Autodesk Inventor part; units mm, degrees
ref_plane "YZ Plane" through (0, 0, 0) normal (1, 0, 0) x (0, 1, 0)
ref_plane "XZ Plane" through (0, 0, 0) normal (0, 1, 0) x (-1, 0, 0)
ref_plane "XY Plane" through (0, 0, 0) normal (0, 0, 1) x (1, 0, 0)
sketch "Sketch1" plane through (0, 0, 0) normal (0, 1, 0) x (-1, 0, 0)
  line L0 (0, 0) -> (161, 0)
  line L1 (161, 0) -> (161, -140)
  line L2 (161, -140) -> (0, -140)
  line L3 (0, -140) -> (0, 0)
  line L4 (156, -135) -> (156, -5)
  line L5 (156, -5) -> (5, -5)
  line L6 (5, -5) -> (5, -135)
  line L7 (5, -135) -> (156, -135)
  dimension "d28" = 151
  dimension "d29" = 130
  dimension "d30" = 5
extrude "Extrusion1" add sketch "Sketch1" along normal blind 44.45
sketch "Sketch2" plane through (0, 0, 0) normal (0, -1, 0) x (1, 0, 0)
  line L0 (-176, 10.75) -> (-5, 10.75)
  line L1 (-5, -150.75) -> (-176, -150.75)
  line L2 (-176, -150.75) -> (-176, 10.75)
  line L3 (-161, 0) -> (0, 0)
  line L4 (0, -140) -> (-161, -140)
  line L5 (-161, -140) -> (-161, 0)
  line L6 (0, -140) -> (-161, -140)
  line L7 (0, 0) -> (0, -140)
  line L8 (-161, 0) -> (0, 0)
  line L9 (-161, -140) -> (-161, 0)
  line L10 (-156, -135) -> (-5, -135)
  line L11 (-156, -5) -> (-156, -135)
  line L12 (-5, -5) -> (-156, -5)
  line L13 (-5, -135) -> (-5, -5)
  line L14 (-5, 10.75) -> (-5, -5)
  line L15 (-5, -135) -> (-5, -150.75)
  dimension "d31" = 161.5
  dimension "d32" = 171
extrude "Extrusion2" add sketch "Sketch2" along normal blind 4 contours L0 L14 L3 L5 L4 L15 L1 L2 | L14 L12 L11 L10 L15 L4 L5 L3
chamfer "Chamfer1" distance 8.5 angle 45 2 edges at (-176, -2, 10.75) (-176, -2, -150.75)
sketch "Sketch3" plane through (0, 0, 0) normal (0, 1, 0) x (1, 0, 0)
  circle A0 centre (-169.6287, -4.3787) radius 1.25
  circle A1 centre (-37.5, -7.75) radius 1.25
  circle A2 centre (-173, 70) radius 1.25
  circle A3 centre (-169.6287, 144.3787) radius 1.25
  circle A4 centre (-37.5, 147.75) radius 1.25
  line L0 (-176, -10.75) -> (-176, 150.75)
  line L1 (-5, -10.75) -> (-176, -10.75)
  line L2 (-176, 150.75) -> (-5, 150.75)
  line L3 (-161, 123.75) -> (-168, 123.75)
  line L4 (-168, 123.75) -> (-168, 103.75)
  line L5 (-168, 103.75) -> (-161, 103.75)
  line L6 (-161, 103.75) -> (-161, 123.75)
  line L7 (-167.5, -10.75) -> (-176, -2.25)
  line L8 (-176, 142.25) -> (-167.5, 150.75)
  line L9 (-171.75, -6.5) -> (-169.6287, -4.3787) construction
  line L10 (-171.75, 146.5) -> (-169.6287, 144.3787) construction
  point P0 (0, 0)
  point P1 (-176, 70)
  point P2 (-176, 70)
  point P3 (-164.5, 103.75)
  point P4 (-164.5, 123.75)
  point P5 (-168, 113.75)
  point P6 (-161, 113.75)
  dimension "d10" = 2.5
  dimension "d11" = 2.5
  dimension "d12" = 2.5
  dimension "d13" = 2.5
  dimension "d14" = 2.5
  dimension "d33" = 138.5
  dimension "d35" = 3
  dimension "d37" = 3
  dimension "d38" = 3
  dimension "d58" = 3
  dimension "d59" = 3
  dimension "d60" = 20
  dimension "d61" = 7
  dimension "d62" = 8
  dimension "d63" = 27
extrude "Extrusion3" cut sketch "Sketch3" against normal blind 11.1125 contours A0 | A1 | A2 | A3 | A4 | L6 L5 L4 L3
sketch "Sketch4" plane through (0, 44.45, 0) normal (0, 1, 0) x (1, 0, 0)
  circle A0 centre (-2.5, 100.75) radius 1
  circle A1 centre (-2.5, 39.25) radius 1
  line L0 (-161, 0) -> (0, 0)
  line L1 (0, 140) -> (-161, 140)
  line L2 (0, 140) -> (-5, 140)
  line L3 (-167.5, 150.75) -> (-5, 150.75)
  line L4 (-5, -10.75) -> (-167.5, -10.75)
  point P0 (-2.5, 140)
  dimension "d20" = 2
  dimension "d39" = 50
  dimension "d51" = 50
extrude "Extrusion4" cut sketch "Sketch4" against normal blind 65.0875
chamfer "Chamfer2" distance 4 angle 45 2 edges at (-83, 0, 0) (-83, 0, -140)
chamfer "Chamfer3" distance 6 angle 45 2 edges at (-161, 0, -51.875) (-161, 0, -131.875)
sketch "Sketch6" plane through (0, 0, 0) normal (1, 0, 0) x (0, 0, -1)
  line L0 (105, 26) -> (125, 26)
  line L1 (125, 26) -> (125, 11)
  line L2 (125, 11) -> (105, 11)
  line L3 (105, 11) -> (105, 26)
  line L4 (5, -4) -> (-10.75, -4)
  line L5 (0, 0) -> (0, 44.45)
  line L6 (140, 0) -> (140, 44.45)
  point P0 (125, 18.5)
  point P1 (105, 18.5)
  dimension "d64" = 15
  dimension "d65" = 15
  dimension "d66" = 20
  dimension "d70" = 15
extrude "Extrusion6" cut sketch "Sketch6" against normal blind 9.05
equation "\"d11\" = d10"
equation "\"d12\" = d11"
equation "\"d13\" = d12"
equation "\"d14\" = d12"
equation "\"d35\" = d34"
equation "\"d37\" = d36"
equation "\"d38\" = d34"
equation "\"d36\" = d34"
properties part number "battery holder"
CAD build for the part. Positions are in the model's coordinates, mm. A direction names the side the tool comes from. Coordinates: 2 decimals unless noted, no trailing zeros. Write each loop counter-clockwise with the first axis right and the second up, starting at its lowest first coordinate (ties: lowest second). Pieces come first, ordered by that corner, then holes. Notation, with made-up numbers: M 51.5,62.25 L 96.5,62.25 A23 cw 96.5,86.25 Z; hole C 74.25,5 d1. An arc over 180 degrees is marked long. Answer as a JSON object with one key per item and string values. Group by question number.
1) Pin check, flat tips, straight feed: pin 1 Ø9 at (y, z) = (1, 6) entering from +X; pin 2 Ø14.5 at (x, y) = (-81.5, 30) entering from -Z; pin 3 Ø1.5 at (x, z) = (-2, -113.5) entering from -Y. Stop position of each tip, or through.
2) Saw through at B-B (x = -63). Write the cut outline in (y, z).
3) Tool access for faces 1 (the face through (-2, 19, -125)), 2 (the face through (-82, 20, -5)), 3 (the face through (-173, 0, -76)), 4 (the face through (-171.81, -2.03, 6.44)): list every direction of +Z, -Z, +X, -X, +Y, -Y with a clear straight run to the whole face (end or side of a thin tool).
4) Mould opens along Z. For faces 5 (the face through (-85, 2, -142)), 6 (the face through (-79, 20, -135)), 7 (the face through (-87, 2, 2)) say: +Z half, -Z half, draft (parallel to the pull), parting line (faces both ways), or undercut.
5) Wall check: line 1 (Z direction, x = -37.5, y = -2.7); line 2 (Z direction, x = -22, y = 32); line 3 (X direction, y = 34, z = -67.5). Give the ranges that are in metal, low to high. Write a range as from..to.
6) Saw through at A-A (z = -79). Write the cut outline in (x, y).
7) Saw through at C-C (y = 29). Write the cut outline in (x, z), plus the area to 3 significant figures.
Values follow:
{
 "1": {"pin 1": "stops at x = -5", "pin 2": "stops at z = -140", "pin 3": "stops at y = 0"},
 "2": {"outline": "M -4,-150.75 L 0,-150.75 L 0,-144 L 4,-140 L 44.45,-140 L 44.45,-135 L -4,-135 Z; M -4,-5 L 44.45,-5 L 44.45,0 L 4,0 L 0,4 L 0,10.75 L -4,10.75 Z"},
 "3": {"face 1": "+X", "face 2": "+Y, -Y", "face 3": "-X, +Y", "face 4": "+Z, -X, +Y, -Y"},
 "4": {"face 5": "-Z half", "face 6": "undercut", "face 7": "+Z half"},
 "5": {"line 1": "z = -150.75..-149, -146.5..-135, -5..6.5, 9..10.75", "line 2": "z = -140..-135, -5..0", "line 3": "x = -161..-156, -5..0"},
 "6": {"outline": "M -176,-4 L -156,-4 L -156,44.45 L -161,44.45 L -161,6 L -167,0 L -176,0 Z; M -5,0 L 0,0 L 0,44.45 L -5,44.45 Z"},
 "7": {"outline": "M -161,-140 L 0,-140 L 0,0 L -161,0 Z; hole M -156,-135 L -5,-135 L -5,-5 L -156,-5 Z; hole C -2.5,-100.75 d2; hole C -2.5,-39.25 d2", "area": "2,900 mm2"}
}
